Geometry check sheet. Reference: the model listing, model coordinates, mm. A direction names the side the tool comes from. Give positions to 0.01 mm unless a question says otherwise; leave off trailing zeros. Loops run counter-clockwise (first coordinate to the right, second up) from the corner with the lowest first, then second, coordinate; pieces in that order, holes last. Notation, with made-up numbers: (24.5, 69.25) -> (66.5, 69.25) arc R11 cw to (66.5, 89.25) -> close; hole circle Ø4 at (49.5, -35). An arc over 180 degrees is marked (long way). Answer as a JSON object with one key per item and string values.
from build123d import *

# Parameters (mm, degrees)
F0_R        = 16
F0_R_2      = 12.25
F1_DEPTH    = 10
F2_W        = 11.453170795
F2_H        = 32.4866687879
F3_DEPTH    = 10.001
F4_T1_DEPTH = 27.6008886653
F4_T3_DEPTH = 16.6375565979
F5_W        = 20
F5_H        = 5
F6_DEPTH    = 10
F7_R        = 2.5
F8_DEPTH    = 18.501
F9_R        = 4.99999


# Not quite as in the source:
# - a fillet or chamfer that OpenCascade refuses, or shapes differently, is made with other operations: its cross-section is extruded or revolved along the edge and cut away or added
# - a fillet or chamfer is up to 0.001 mm smaller than in the source, because OpenCascade refuses the exact size


with BuildPart() as f1:
    # F0 (on Top) → F1 (new body)
    with BuildSketch(Plane.XY):
        Circle(F0_R)
        Circle(F0_R_2, mode=Mode.SUBTRACT)
    extrude(amount=F1_DEPTH)

    # F2 (on face) → F3 (cut, through all)
    with BuildSketch(Plane.XY.offset(10)):
        with Locations((-13.3922861423, 0.2399678342)):
            Rectangle(F2_W, F2_H)
    extrude(amount=-F3_DEPTH, mode=Mode.SUBTRACT)

    # F4: fillet of radius 2 on 4 edges, made by hand

    # F4_s2 → F4_t1 (cut)
    with BuildSketch(Plane.XY.offset(-8.8004443327)):
        with BuildLine():
            ThreePointArc((-7.6657007448, 13.0752565967), (-6.7633409093, 11.4033755993), (-4.8705146754, 11.2401328638))
            ThreePointArc((-4.8705146754, 11.2401328638), (-6.3244783193, 10.491114049), (-7.6657007448, 9.5550788637))
            Line((-7.6657007448, 9.5550788637), (-7.6657007448, 13.0752565967))
        make_face()
        with BuildLine():
            ThreePointArc((-4.8705146754, -11.2401328638), (-6.7633409093, -11.4033755993), (-7.6657007448, -13.0752565967))
            Line((-7.6657007448, -13.0752565967), (-7.6657007448, -9.5550788637))
            ThreePointArc((-7.6657007448, -9.5550788637), (-6.3244783193, -10.491114049), (-4.8705146754, -11.2401328638))
        make_face()
    extrude(amount=F4_T1_DEPTH, mode=Mode.SUBTRACT)

    # F4_s4 → F4_t3 (cut)
    with BuildSketch(Plane.XY.offset(-3.318778299)):
        with BuildLine():
            ThreePointArc((-6.4750865655, -14.6312423932), (-7.3418230019, -13.8934897778), (-7.6657007448, -12.8023370941))
            Line((-7.6657007448, -12.8023370941), (-7.6657007448, -14.0441102278))
            ThreePointArc((-7.6657007448, -14.0441102278), (-7.076485532, -14.3500297044), (-6.4750865655, -14.6312423932))
        make_face()
        with BuildLine():
            ThreePointArc((-6.4750865655, 14.6312423932), (-7.3418230019, 13.8934897778), (-7.6657007448, 12.8023370941))
            Line((-7.6657007448, 12.8023370941), (-7.6657007448, 14.0441102278))
            ThreePointArc((-7.6657007448, 14.0441102278), (-7.076485532, 14.3500297044), (-6.4750865655, 14.6312423932))
        make_face()
    extrude(amount=F4_T3_DEPTH, mode=Mode.SUBTRACT)

    # F5 (on face) → F6 (join)
    with BuildSketch(Plane.XY.offset(10)):
        with Locations((23.4022848308, 0)):
            Rectangle(F5_W, F5_H)
    extrude(amount=-F6_DEPTH)

    # F7 (on face) → F8 (cut, through all)
    with BuildSketch(Plane.XZ.offset(2.5)):
        with Locations((28.4022848308, 5)):
            Circle(F7_R)
    extrude(amount=-F8_DEPTH, mode=Mode.SUBTRACT)

    # F9 (radius 5 in the source; OpenCascade refuses exactly that, so slightly less here)
    f9_edges = [f1.edges().sort_by_distance(p)[0] for p in [
        (33.402285, 0, 10),
        (33.402285, 0, 0),
    ]]
    fillet(f9_edges, radius=F9_R)


solid = f1.part
1) Section check D-D on x = 20. Record the cut outline in (y, z), plus the area to 3 significant figures.
Geometry check:
{"outline": "(-2.5, 0) -> (2.5, 0) -> (2.5, 10) -> (-2.5, 10) -> close", "area": "50.0 mm2"}
2) Draft check along Y on faces 4 (the face through (31.899, 0.035, 1.426)), 5 (the face through (23, -2.5, 5)), 6 (the face through (-6.73, 11.38, 4.93)), 7 (the face through (-7.295, 13.962, 4.93)). Enter one of: pulls with the +Y half, pulls with the -Y half, needs draft (parallel to the pull), parting line crosses it, or undercut.
Geometry check:
{"face 4": "needs draft", "face 5": "pulls with the -Y half", "face 6": "undercut", "face 7": "pulls with the +Y half"}
3) Tool access check on faces 1 (the face through (23, 2.5, 5)), 2 (the face through (-6.68, -11.35, 4.93)), 3 (the face through (7.47, -14.15, 4.93)). Record the directions out of +Z, -Z, +X, -X, +Y, -Y that give a thin tool (end or side, any length) a straight path to the whole face; none if there is none.
Geometry check:
{"face 1": "+Z, -Z, +X, +Y", "face 2": "+Z, -Z", "face 3": "+Z, -Z, -Y"}
4) Section check C-C on z = 1.25. Record the cut outline in (x, y).
Geometry check:
{"outline": "(-7.66, -12.94) arc R2 ccw to (-6.48, -14.63) arc R16 ccw to (15.8, -2.5) -> (31.71, -2.5) -> (31.71, 2.5) -> (15.8, 2.5) arc R16 ccw to (-6.48, 14.63) arc R2 ccw to (-7.66, 12.94) arc R2 ccw to (-4.87, 11.24) arc R12.25 cw (long way) to (-4.87, -11.24) arc R2 ccw to start"}
5) Material ranges on line 1 along Y through (x, z) = (0, 5); line 2 along Y through (x, z) = (25.5, 8.75); line 3 along Y through (x, z) = (3, 8.75), recorded low to high. Write a range as from..to.
Geometry check:
{"line 1": "y = -16..-12.25, 12.25..16", "line 2": "y = -2.5..2.5", "line 3": "y = -15.72..-11.88, 11.88..15.72"}
6) Depth check by flat-ended pin: P1, Ø5, axis at x = 28, z = 7.5, coming from the -Y side; P2, Ø3, axis at x = 24, z = 5.5, coming from the +Y side; P3, Ø1, axis at x = 11, z = 7, coming from the -Y side. Enter the tip coordinate at first touch or a pass-through.
Geometry check:
{"P1": "stops at y = -2.5", "P2": "stops at y = 2.5", "P3": "stops at y = -12.07"}
7) Section check A-A on x = 0. Record the cut outline in (y, z).
Geometry check:
{"outline": "(-16, 0) -> (-12.25, 0) -> (-12.25, 10) -> (-16, 10) -> close; (12.25, 0) -> (16, 0) -> (16, 10) -> (12.25, 10) -> close"}
